Source: CAD feature listing. Evaluate the final solid. Frame: model axes, mm. A direction names the side the tool comes from. Coordinates: 2 decimals unless noted, no trailing zeros. Order: outer loops, then holes, each group sorted by start corner. A loop starts at its lowest first (then second) coordinate and runs counter-clockwise, first axis right, second up. Notation, with made-up numbers: (43.5, -11) - (77.5, -11) arc R24 ccw to (77.5, 4) - close; hole circle Ø4 at (76.5, -1.75). An arc over 180 degrees is marked (long way). One line per question, with ' | ' between items. Start each with the question number.
(1) Section A-A (y = 0). Return the cut outline in (x, z) (3 decimals).
(2) Section C-C (y = -79). Return the cut outline in (x, z).
(3) Contact query for flat-ended pins moving along their axis: P1, Ø1, axis at x = -3.5, z = -1, coming from the -Y side; P2, Ø5.5, axis at y = 0, z = 0, coming from the +X side. Output: stop coordinate, or through.
(4) Section D-D (y = 154). Return the cut outline in (x, z), then the cut area to 3 significant figures.
(5) Access query for faces 1 (the flat face through (-3.94, 31.97, -10.03)), 2 (the flat face through (-3.944, -102.92, -8.756)), 3 (the flat face through (-3.94, -31.37, 11.29)). Directions: +Z, -Z, +X, -X, +Y, -Y. A direction counts if a zero-diameter tool reaches every point of the face in a straight line with its end or side. Return the directions, or none.
(6) Draft query along Y for faces 4 (the flat face through (-3.94, -31.97, -10.03)), 5 (the flat face through (-3.944, 162.849, -4.654)), 6 (the flat face through (-3.944, -162.849, -4.654)). Return one class per face: +Y half, -Y half, draft (parallel to the pull), parting line (faces both ways), or undercut.
(7) Line query: line 1 along Y through (x, z) = (-5, 0) (3 decimals); line 2 along Z through (x, y) = (-3.5, 0) (3 decimals); line 3 along Y through (x, z) = (-4, -0.75). Output: solid intervals per line, ascending.
from build123d import *

# Parameters (mm, degrees)
BOSS_EXTRUDE1_DEPTH     = 8
BOSS_EXTRUDE1_2_DEPTH   = 8
SKETCH2_R               = 12
BOSS_EXTRUDE2_DEPTH     = 8
CUT_EXTRUDE1_DEPTH      = 179.583327588
CUT_EXTRUDE1_DEPTH_BACK = 179.583327588
SKETCH3_R               = 3.175


with BuildPart() as part:
    # Sketch1 → Boss-Extrude1 (new body)
    with BuildSketch(Plane(origin=(0, 0, 0), x_dir=(0, 0, -1), z_dir=(1, 0, 0))):
        Polygon((-8.001, 10), (-14.6685, 53.34), (-6.8453, 151.13), (-2.4892, 174.244), (0, 177.8), (3.7338, 174.244), (5.6007, 151.13), (12.0015, 53.34), (8.001, 10), align=None)
    extrude(amount=-BOSS_EXTRUDE1_DEPTH)



with BuildPart() as body_2:
    # Sketch1 → Boss-Extrude1 2 (new body)
    with BuildSketch(Plane(origin=(0, 0, 0), x_dir=(0, 0, -1), z_dir=(1, 0, 0))):
        Polygon((-8.001, -10), (-14.6685, -53.34), (-6.8453, -151.13), (-2.4892, -174.244), (0, -177.8), (3.7338, -174.244), (5.6007, -151.13), (12.0015, -53.34), (8.001, -10), align=None)
    extrude(amount=-BOSS_EXTRUDE1_2_DEPTH)


with BuildPart() as part_1:
    add(part.part)

    add(body_2.part)  # Boss-Extrude2 merges body 2
    # Sketch2 → Boss-Extrude2 (add)
    with BuildSketch(Plane(origin=(0, 0, 0), x_dir=(0, 0, -1), z_dir=(1, 0, 0))):
        Circle(SKETCH2_R)
    extrude(amount=-BOSS_EXTRUDE2_DEPTH)

    # Sketch3 → Cut-Extrude1 (cut, two sides: drawn at the far end of the back side and taken through both)
    with BuildSketch(Plane(origin=(0, 0, 0), x_dir=(0, 0, -1), z_dir=(1, 0, 0)).offset(-CUT_EXTRUDE1_DEPTH_BACK)):
        Circle(SKETCH3_R)
    extrude(amount=CUT_EXTRUDE1_DEPTH + CUT_EXTRUDE1_DEPTH_BACK, mode=Mode.SUBTRACT)


solid = part_1.part
Response values:
1) outline: (-8, -12) - (0, -12) - (0, -3.175) - (-8, -3.175) - close; (-8, 3.175) - (0, 3.175) - (0, 12) - (-8, 12) - close
2) outline: (-8, -10.32) - (0, -10.32) - (0, 12.62) - (-8, 12.62) - close
3) P1: stops at y = -177.32 | P2: passes through
4) outline: (-8, -5.37) - (0, -5.37) - (0, 6.3) - (-8, 6.3) - close | area: 93.4 mm²
5) face 1: -Z, +X, -X | face 2: -Z, +X, -X, -Y | face 3: +Z, +X, -X
6) face 4: undercut | face 5: +Y half | face 6: -Y half
7) line 1: y = -177.8 to -3.175, 3.175 to 177.8 | line 2: z = -12 to -3.175, 3.175 to 12 | line 3: y = -177.09 to -3.09, 3.09 to 177.09
